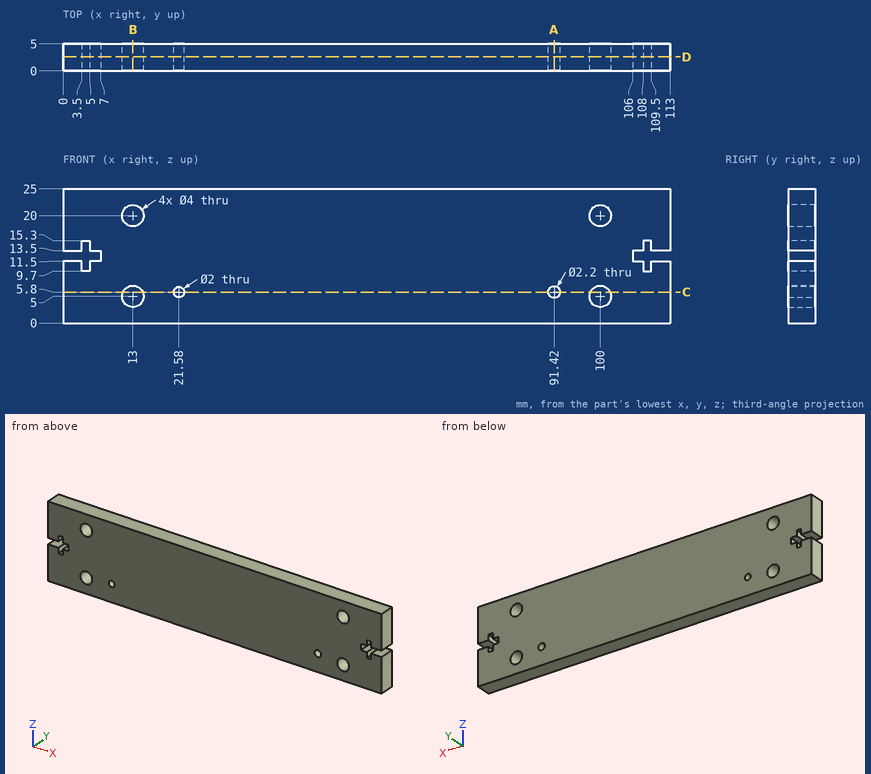
Could you check a few things on this drawing? It's one solid part, dimensions in mm from its lowest x, y, z. Coordinates: 2 decimals unless noted, no trailing zeros. Write each loop counter-clockwise with the first axis right and the second up, starting at its lowest first coordinate (ties: lowest second). Pieces come first, ordered by that corner, then holes. Notation, with made-up numbers: (49.5, -23) - (88.5, -23) arc R18 ccw to (88.5, 0) - close; hole circle Ø5 at (57, -2.75). An arc over 180 degrees is marked (long way). Return JSON: item names as keys, results as strings. Group by question number.
Item 1: I'm going to push flat-ended pins straight in: pin 1 Ø2 at (x, y) = (101.5, 3) entering from -Z; pin 2 Ø0.6 at (y, z) = (3, 12) entering from -X. Where does each tip first touch, or does it pass through?
Item 2: If we section it at A-A (x = 91.42): Write out the boundary of the cut face in (y, z).
Item 3: Please list where these lines run through material, in increasing order: probe 1 along Z at (x, y) = (100, 1.95); probe 2 along X at (y, z) = (2.05, 6.5); probe 3 along X at (y, z) = (1.5, 4).
Item 4: If we section it at B-B (x = 13): Write out the boundary of the cut face in (y, z), then the cut area to 3 significant figures.
Item 5: If we section it at D-D (y = 2.6): Count the separate pieces of the cut face and the enclosed holes in it, then the cut area to 3 significant figures.
Item 6: If we section it at C-C (z = 5.8): Write out the boundary of the cut face in (x, y).
Return value:
{
 "1": {"pin 1": "stops at z = 0", "pin 2": "stops at x = 7"},
 "2": {"outline": "(0, 0) - (5, 0) - (5, 4.7) - (0, 4.7) - close; (0, 6.9) - (5, 6.9) - (5, 25) - (0, 25) - close"},
 "3": {"probe 1": "z = 0 to 3, 7 to 18, 22 to 25", "probe 2": "x = 0 to 11.68, 14.32 to 20.87, 22.29 to 90.57, 92.27 to 98.68, 101.32 to 113", "probe 3": "x = 0 to 11.27, 14.73 to 98.27, 101.73 to 113"},
 "4": {"outline": "(0, 0) - (5, 0) - (5, 3) - (0, 3) - close; (0, 7) - (5, 7) - (5, 18) - (0, 18) - close; (0, 22) - (5, 22) - (5, 25) - (0, 25) - close", "area": "85.0 mm^2"},
 "5": {"separate pieces": "1", "enclosed holes": "6", "area": "2,730 mm^2"},
 "6": {"outline": "(0, 0) - (11.17, 0) - (11.17, 5) - (0, 5) - close; (14.83, 0) - (20.58, 0) - (20.58, 5) - (14.83, 5) - close; (22.58, 0) - (90.32, 0) - (90.32, 5) - (22.58, 5) - close; (92.52, 0) - (98.17, 0) - (98.17, 5) - (92.52, 5) - close; (101.83, 0) - (113, 0) - (113, 5) - (101.83, 5) - close"}
}
